Autodesk Inventor part; units mm, degrees
ref_plane "YZ Plane" through (0, 0, 0) normal (1, 0, 0) x (0, 1, 0)
ref_plane "XZ Plane" through (0, 0, 0) normal (0, 1, 0) x (-1, 0, 0)
ref_plane "XY Plane" through (0, 0, 0) normal (0, 0, 1) x (1, 0, 0)
sketch "Sketch1" plane through (0, 0, 0) normal (0, 1, 0) x (-1, 0, 0)
  circle A0 centre (0, 0) radius 3.2512
  line L0 (6.35, 6.35) -> (-6.35, 6.35)
  line L1 (-6.35, 6.35) -> (-6.35, -12.7)
  line L2 (-6.35, -12.7) -> (6.35, -12.7)
  line L3 (6.35, -12.7) -> (6.35, 6.35)
  point P0 (0, 6.35)
  dimension "d0" = 6.5024
  dimension "d1" = 12.7
  dimension "d2" = 19.05
  dimension "d3" = 6.35
extrude "Extrusion1" add sketch "Sketch1" along normal blind 3.175
sketch "Sketch2" plane through (0, 3.175, 0) normal (0, 1, 0) x (1, 0, 0)
  line L0 (6.35, 12.7) -> (-6.35, 12.7)
  line L1 (6.35, -6.35) -> (6.35, 12.7)
  line L2 (-6.35, 12.7) -> (6.35, 12.7)
  line L3 (6.35, 12.7) -> (6.35, 6.35)
  line L4 (6.35, 6.35) -> (-6.35, 6.35)
  line L5 (-6.35, 6.35) -> (-6.35, 12.7)
  point P0 (0, 0)
  dimension "d6" = 6.35
extrude "Extrusion2" add sketch "Sketch2" along normal blind 6.35
sketch "Sketch3" plane through (6.35, 0, -12.7) normal (0, 0, -1) x (-1, 0, 0)
  circle A0 centre (6.35, 4.7625) radius 3.175
  line L0 (12.7, 0) -> (12.7, 9.525)
  line L1 (0, 9.525) -> (12.7, 9.525)
  point P0 (6.35, 0)
  point P1 (12.7, 4.7625)
  point P2 (6.35, 9.525)
  dimension "d9" = 6.35
extrude "Extrusion3" cut sketch "Sketch3" against normal up to surface (6.35 mm away)
properties part number "OUTK_022_BadPivot" material "Aluminum 6061"
Read the model definition and answer for the solid it produces. Units are mm, in the model's axes. A direction names the side the tool comes from. Round coordinates to 2 decimals unless told otherwise and drop trailing zeros. Write each loop counter-clockwise with the first axis right and the second up, starting at its lowest first coordinate (ties: lowest second). Pieces come first, ordered by that corner, then holes. Notation, with made-up numbers: M 66.25,57.5 L 81.25,57.5 A17 cw 81.25,62.5 Z; hole C 11,78.25 d6. An arc over 180 degrees is marked long. One line per item, written item: value.
Q1. Find section A-A on x = -0.25. Write down the section's boundary in (y, z) (3 decimals), plus the area to 3 significant figures.
Data:
outline: M 0,-12.7 L 1.597,-12.7 L 1.597,-6.35 L 3.175,-6.35 L 3.175,-3.242 L 0,-3.242 Z; M 0,3.242 L 3.175,3.242 L 3.175,6.35 L 0,6.35 Z; M 7.928,-12.7 L 9.525,-12.7 L 9.525,-6.35 L 7.928,-6.35 Z
area: 40.0 mm2
Q2. Find section C-C on z = 0. Write down the section's boundary in (x, y) (3 decimals), plus the area to 3 significant figures.
Data:
outline: M -6.35,0 L -3.251,0 L -3.251,3.175 L -6.35,3.175 Z; M 3.251,0 L 6.35,0 L 6.35,3.175 L 3.251,3.175 Z
area: 19.7 mm2
Q3. Straight lines are drawn through the part: line 1 (Y direction, x = 0, z = -11.5) (1 decimal); line 2 (Z direction, x = 0, y = 1.85); line 3 (Y direction, x = -1, z = -4.25) (3 decimals). For each, find the intervals that lie inside material, in ascending order. Write a range as [from, to].
Data:
line 1: [0, 1.6], [7.9, 9.5]
line 2: [-6.35, -3.25], [3.25, 6.35]
line 3: [0, 3.175]
Q4. Find section D-D on y = 2. Write down the section's boundary in (x, z) (3 decimals).
Data:
outline: M -6.35,-12.7 L -1.565,-12.7 L -1.565,-6.35 L 1.565,-6.35 L 1.565,-12.7 L 6.35,-12.7 L 6.35,6.35 L -6.35,6.35 Z; hole C 0,0 d6.502
Q5. Which of the six approach directions +Z, -Z, +X, -X, +Y, -Y give full straight-line access (tool end or side, diameter ignored) to faces 4 (the flat face through (2, 3.175, 3)), 5 (the cylindrical face through (0.688, 1.663, -9.569)), 6 (the flat face through (6.35, 3, -5))?
Data:
face 4: +Z, +X, -X, +Y
face 5: -Z
face 6: +Z, -Z, +X, +Y, -Y
Q6. Find section B-B on y = 5. Write down the section's boundary in (x, z), plus the area to 3 significant figures.
Data:
outline: M -6.35,-12.7 L -3.17,-12.7 L -3.17,-6.35 L -6.35,-6.35 Z; M 3.17,-12.7 L 6.35,-12.7 L 6.35,-6.35 L 3.17,-6.35 Z
area: 40.4 mm2
Q7. For a pull along Y with two mould halves and no side action, classify faces 1 (the flat face through (0, 9.525, -10)), 2 (the flat face through (0, 3, -6.35)), 3 (the flat face through (-1.3, 1.5, -12.7)) as +Y half, -Y half, draft (parallel to the pull), parting line (faces both ways), or undercut.
Data:
face 1: +Y half
face 2: undercut
face 3: draft
Q8. Flat-ended cylindrical pins translate along their axes: pin 1 Ø3 at (x, y) = (4, 6.5) entering from +Z; pin 2 Ø1 at (x, z) = (1.5, -3.5) entering from +Y (3 decimals); pin 3 Ø0.5 at (x, y) = (0, 2.5) entering from -Z. Find the tip coordinate at first contact, or state that the pin passes through.
Data:
pin 1: z = -6.35
pin 2: y = 3.175
pin 3: z = -6.35
